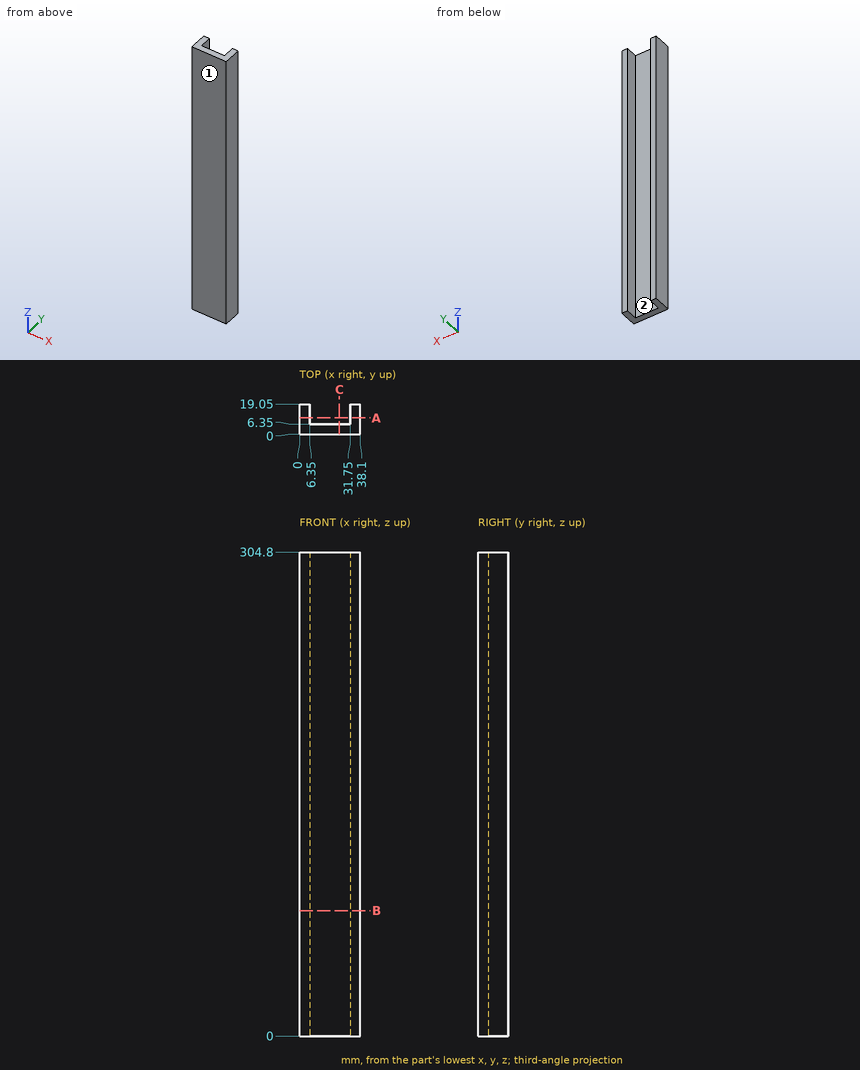
Input: dimensioned drawing with shaded views. Units: mm. Origin: part minimum x, y, z. A direction names the side the tool comes from. Give positions to 0.01 mm unless a question says otherwise; leave off trailing zeros. Order: outer loops, then holes, each group sorted by start corner. A loop starts at its lowest first (then second) coordinate and runs counter-clockwise, first axis right, second up. Notation, with made-up numbers: (69, 22) -> (89, 22) arc R25 ccw to (89, 50) -> close; hole circle Ø7 at (21.25, -25). An arc over 180 degrees is marked (long way). Use a Markdown table: item, result.
1) Section query A-A, the plane y = 10.25. Return the cut outline in (x, z), then the cut area to 3 significant figures.
Answer list:
| item | result |
|---|---|
| outline | (0, 0) -> (6.35, 0) -> (6.35, 304.8) -> (0, 304.8) -> close; (31.75, 0) -> (38.1, 0) -> (38.1, 304.8) -> (31.75, 304.8) -> close |
| area | 3,870 mm² |
2) Section query C-C, the plane x = 25. Return the cut outline in (y, z).
Answer list:
| item | result |
|---|---|
| outline | (0, 0) -> (6.35, 0) -> (6.35, 304.8) -> (0, 304.8) -> close |
3) Section query B-B, the plane z = 79. Return the cut outline in (x, y), then the cut area to 3 significant figures.
Answer list:
| item | result |
|---|---|
| outline | (0, 0) -> (38.1, 0) -> (38.1, 19.05) -> (31.75, 19.05) -> (31.75, 6.35) -> (6.35, 6.35) -> (6.35, 19.05) -> (0, 19.05) -> close |
| area | 403 mm² |
4) Reachability of the marked faces 1 and 2 from +Z, -Z, +X, -X, +Y, -Y: full face, straight path, thin tool, end or side. Return the list, or none.
Answer list:
| item | result |
|---|---|
| face 1 | +Z, -Z, +X, -X, -Y |
| face 2 | +Z, -Z, +Y |
5) Ray query, line 1 along X through (y, z) = (13, 28.5); line 2 along Y through (x, z) = (6.5, 249.5). Return the intervals inside material, ascending. Write a range as [from, to].
Answer list:
| item | result |
|---|---|
| line 1 | [0, 6.35], [31.75, 38.1] |
| line 2 | [0, 6.35] |
6) Contact query for flat-ended pins moving along their axis: P1, Ø5, axis at x = 22, z = 222, coming from the -Y side; P2, Ø12.5, axis at x = 17.5, z = 227.5, coming from the +Y side. Output: stop coordinate, or through.
Answer list:
| item | result |
|---|---|
| P1 | y = 0 |
| P2 | y = 6.35 |
